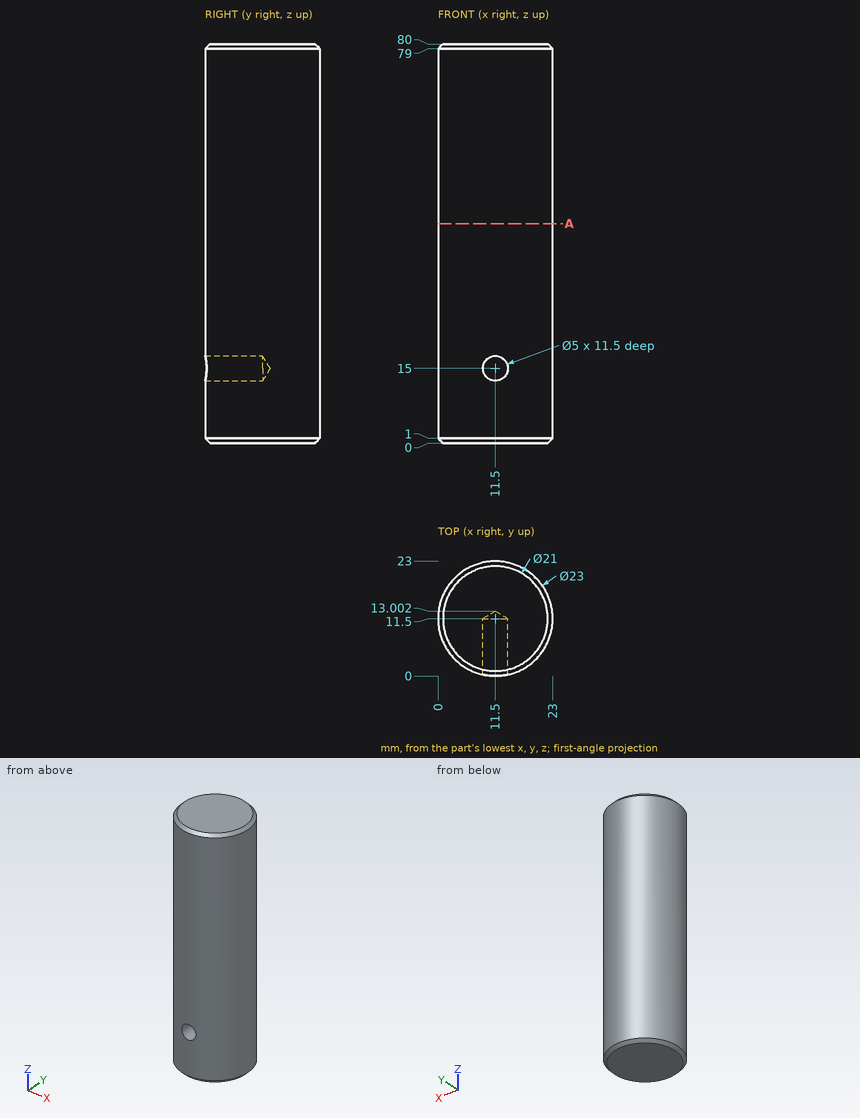
Part print with two shaded views. Sizes in mm from the minimum x, y, z corner. Round coordinates to 2 decimals unless told otherwise and drop trailing zeros. Order: outer loops, then holes, each group sorted by start corner. A loop starts at its lowest first (then second) coordinate and runs counter-clockwise, first axis right, second up. Notation, with made-up numbers: M 60,43.5 L 103,43.5 A25 cw 103,63.5 Z; hole C 31.5,87 d11. An arc over 180 degrees is marked long. Answer in a Markdown table with one row per item. Add a question column.
Q1. Cut at A-A on z = 44. Give the cut face in (x, y).
Q2. Wall check: L1, parallel to Z at x = 11.5, y = 7.5; L2, parallel to X at y = 8.75, z = 15; L3, parallel to X at y = 4, z = 15. Give the ranges that are in metal, low to high. Write a range as from..to.
Q3. Pin check, flat tips, straight feed: pin 1 (8 mm diameter, centred on x = 4, z = 43, fed in from +Y); pin 2 (5 mm diameter, centred on y = 16.5, z = 48.5, fed in from -X) (3 decimals); pin 3 (8 mm diameter, centred on y = 5.5, z = 58, fed in from +X) (1 decimal). Stop position of each tip, or through.
Established:
| question | item | result |
|---|---|---|
| 1 | outline | C 11.5,11.5 d23 |
| 2 | L1 | z = 0..12.5, 17.5..80 |
| 2 | L2 | x = 0.33..9, 14..22.67 |
| 2 | L3 | x = 2.78..9, 14..20.22 |
| 3 | pin 1 | stops at y = 22.45 |
| 3 | pin 2 | stops at x = 0.275 |
| 3 | pin 3 | stops at x = 22.8 |
